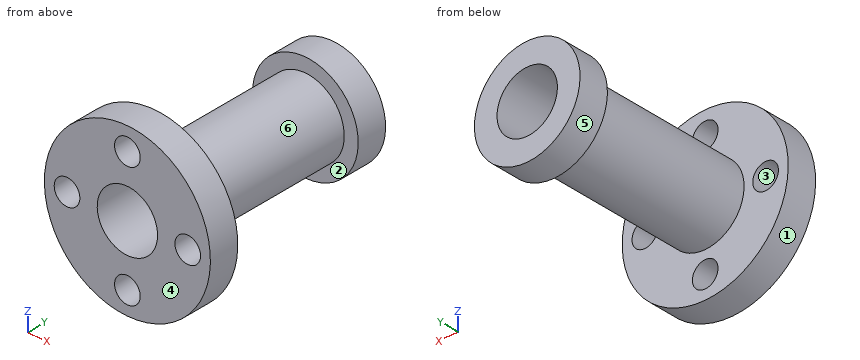
from build123d import *

# Parameters (mm, degrees)
M3_CLEARANCE_HOLE1_REACH  = 35.793
M3_CLEARANCE_HOLE1_BORE_R = 1.7


with BuildPart() as part:
    # Sketch2 → Revolve1 (revolve)
    with BuildSketch(Plane.XY, mode=Mode.PRIVATE) as revolve1_sk:
        Polygon((4, 30), (4, 0), (11, 0), (11, 4), (5.15, 4), (5.15, 26), (7, 26), (7, 30), align=None)
    revolve(revolve1_sk.sketch.rotate(Axis((0, 0, 0), (0, 1, 0)), 90), axis=Axis((0, 0, 0), (0, 1, 0)))

    # M3 Clearance Hole1 bore → M3 Clearance Hole1 (cut, up to next)
    with BuildSketch(Plane(origin=(0, 0, 0), x_dir=(-1, 0, 0), z_dir=(0, -1, 0)), mode=Mode.PRIVATE) as m3_clearance_hole1_sk1:
        with Locations((0, -8)):
            Circle(M3_CLEARANCE_HOLE1_BORE_R)
    m3_clearance_hole1_tool1 = extrude(m3_clearance_hole1_sk1.sketch, amount=-M3_CLEARANCE_HOLE1_REACH, mode=Mode.PRIVATE) & part.part
    # M3 Clearance Hole1 bore → M3 Clearance Hole1 (cut, up to next)
    with BuildSketch(Plane(origin=(0, 0, 0), x_dir=(-1, 0, 0), z_dir=(0, -1, 0)), mode=Mode.PRIVATE) as m3_clearance_hole1_sk2:
        with Locations((-8, 0)):
            Circle(M3_CLEARANCE_HOLE1_BORE_R)
    m3_clearance_hole1_tool2 = extrude(m3_clearance_hole1_sk2.sketch, amount=-M3_CLEARANCE_HOLE1_REACH, mode=Mode.PRIVATE) & part.part
    # M3 Clearance Hole1 bore → M3 Clearance Hole1 (cut, up to next)
    with BuildSketch(Plane(origin=(0, 0, 0), x_dir=(-1, 0, 0), z_dir=(0, -1, 0)), mode=Mode.PRIVATE) as m3_clearance_hole1_sk3:
        with Locations((0, 8)):
            Circle(M3_CLEARANCE_HOLE1_BORE_R)
    m3_clearance_hole1_tool3 = extrude(m3_clearance_hole1_sk3.sketch, amount=-M3_CLEARANCE_HOLE1_REACH, mode=Mode.PRIVATE) & part.part
    # M3 Clearance Hole1 bore → M3 Clearance Hole1 (cut, up to next)
    with BuildSketch(Plane(origin=(0, 0, 0), x_dir=(-1, 0, 0), z_dir=(0, -1, 0)), mode=Mode.PRIVATE) as m3_clearance_hole1_sk4:
        with Locations((8, 0)):
            Circle(M3_CLEARANCE_HOLE1_BORE_R)
    m3_clearance_hole1_tool4 = extrude(m3_clearance_hole1_sk4.sketch, amount=-M3_CLEARANCE_HOLE1_REACH, mode=Mode.PRIVATE) & part.part
    add(m3_clearance_hole1_tool1.solids().sort_by_distance((0, 0, 8))[0], mode=Mode.SUBTRACT)
    add(m3_clearance_hole1_tool2.solids().sort_by_distance((8, 0, 0))[0], mode=Mode.SUBTRACT)
    add(m3_clearance_hole1_tool3.solids().sort_by_distance((0, 0, -8))[0], mode=Mode.SUBTRACT)
    add(m3_clearance_hole1_tool4.solids().sort_by_distance((-8, 0, 0))[0], mode=Mode.SUBTRACT)


solid = part.part
Could you check a few things on this model? Use its own coordinates, in mm. Face numbers are marked on the shaded views. A direction names the side the tool comes from. Round coordinates to 2 decimals unless told otherwise and drop trailing zeros. Loops run counter-clockwise (first coordinate to the right, second up) from the corner with the lowest first, then second, coordinate; pieces in that order, holes last. Notation, with made-up numbers: (37, 21.25) - (96, 21.25) arc R22 ccw to (96, 57.25) - close; hole circle Ø4 at (-29.75, 23.5). An arc over 180 degrees is marked (long way). Write item = value, one per line.
1) On a 3-axis mill with a long thin cutter (end or side, diameter ignored), from which of +Z, -Z, +X, -X, +Y, -Y can I reach the whole of each face in a straight line? I mean the marked faces 1, 2 and 3. Say none if no direction works.
Computed:
face_1 = +Y, -Y
face_2 = none
face_3 = -Y
2) Imagine slicing it at D-D (x = 0). Please give me the cut outline in (y, z).
Computed:
outline = (0, -11) - (4, -11) - (4, -9.7) - (0, -9.7) - close; (0, -6.3) - (4, -6.3) - (4, -5.15) - (26, -5.15) - (26, -7) - (30, -7) - (30, -4) - (0, -4) - close; (0, 4) - (30, 4) - (30, 7) - (26, 7) - (26, 5.15) - (4, 5.15) - (4, 6.3) - (0, 6.3) - close; (0, 9.7) - (4, 9.7) - (4, 11) - (0, 11) - close
3) I need wall thicknesses on line 1 along X through (y, z) = (2.9, 0); line 2 along Y through (x, z) = (5.75, -1); line 3 along Y through (x, z) = (0.25, -6.5). Which ranges of each line are inside material? Lowest first, please. Write a range as from..to.
Computed:
line_1 = -11..-9.7, -6.3..-4, 4..6.3, 9.7..11
line_2 = 0..4, 26..30
line_3 = 26..30
4) If we mould it in two halves opening along Y, with no side actions, what happens to the marked faces 4, 5 and 6? For each: pulls with the +Y half, pulls with the -Y half, needs draft (parallel to the pull), parting line crosses it, or undercut.
Computed:
face_4 = pulls with the -Y half
face_5 = needs draft
face_6 = undercut
5) Imagine slicing it at A-A (z = 0). Please give me the cut outline in (x, y).
Computed:
outline = (-11, 0) - (-9.7, 0) - (-9.7, 4) - (-11, 4) - close; (-7, 26) - (-5.15, 26) - (-5.15, 4) - (-6.3, 4) - (-6.3, 0) - (-4, 0) - (-4, 30) - (-7, 30) - close; (4, 0) - (6.3, 0) - (6.3, 4) - (5.15, 4) - (5.15, 26) - (7, 26) - (7, 30) - (4, 30) - close; (9.7, 0) - (11, 0) - (11, 4) - (9.7, 4) - close
6) I'm going to push flat-ended pins straight in: P1, Ø10, axis at x = 3, y = 26.5, coming from the +Z side; P2, Ø4, axis at x = 0, z = -8, coming from the +Y side; P3, Ø8, axis at y = 5, z = -7.5, coming from the +X side; P4, Ø3, axis at x = 4.5, y = 26, coming from the -Z side. Where does each tip first touch, or does it pass through?
Computed:
P1 = 7
P2 = 30
P3 = 10.38
P4 = -6.32
7) Imagine slicing it at B-B (x = -8). Please give me the cut outline in (y, z), and give its area (3 significant figures).
Computed:
outline = (0, -7.55) - (4, -7.55) - (4, -1.7) - (0, -1.7) - close; (0, 1.7) - (4, 1.7) - (4, 7.55) - (0, 7.55) - close
area = 46.8 mm2
8) Imagine slicing it at C-C (z = -2.25). Please give me the cut outline in (x, y).
Computed:
outline = (-10.77, 0) - (-3.31, 0) - (-3.31, 30) - (-6.63, 30) - (-6.63, 26) - (-4.63, 26) - (-4.63, 4) - (-10.77, 4) - close; (3.31, 0) - (10.77, 0) - (10.77, 4) - (4.63, 4) - (4.63, 26) - (6.63, 26) - (6.63, 30) - (3.31, 30) - close
